```python
from build123d import *

# Parameters (mm, degrees)
F0_W     = 209.55
F0_H     = 165.1
F1_DEPTH = 3.175
F2_W     = 6.35
F2_H     = 38.1
F2_W_2   = 38.1
F2_H_2   = 6.35
F3_DEPTH = 25.4
F4_W     = 25.4
F4_H     = 50.8
F4_W_2   = 38.1
F5_DEPTH = 25.4


# Not quite as in the source:
# - a length typed as a fraction of an inch, garbled in the dataset ("3 / 203.2 mm" for 3/8 in), is restored


with BuildPart() as f1:
    # F0 (on Top) → F1 (new body)
    with BuildSketch(Plane.XY):
        Rectangle(F0_W, F0_H)
    extrude(amount=F1_DEPTH)

    # F2 (on face) → F3 (cut)
    with BuildSketch(Plane.XY.offset(3.175)):
        with Locations((-101.6, 38.1)):
            Rectangle(F2_W, F2_H)
        with Locations((-101.6, -38.1)):
            Rectangle(F2_W, F2_H)
        with Locations((101.6, 38.1)):
            Rectangle(F2_W, F2_H)
        with Locations((101.6, -38.1)):
            Rectangle(F2_W, F2_H)
        with Locations((-41.275, -79.375)):
            Rectangle(F2_W_2, F2_H_2)
        with Locations((41.275, -79.375)):
            Rectangle(F2_W_2, F2_H_2)
        with Locations((41.275, 79.375)):
            Rectangle(F2_W_2, F2_H_2)
        with Locations((-41.275, 79.375)):
            Rectangle(F2_W_2, F2_H_2)
    extrude(amount=-F3_DEPTH, mode=Mode.SUBTRACT)

    # F4 (on face) → F5 (cut)
    with BuildSketch(Plane.XY.offset(3.175)):
        with Locations((-79.375, -44.45)):
            Rectangle(F4_W, F4_H)
        with Locations((79.375, -44.45)):
            Rectangle(F4_W, F4_H)
        with Locations((0, -44.45)):
            Rectangle(F4_W_2, F4_H)
    extrude(amount=-F5_DEPTH, mode=Mode.SUBTRACT)


solid = f1.part
```
Here's how the part is built. I have some questions about the finished solid (model axes, mm). Coordinates: 2 decimals unless noted, no trailing zeros. Order: outer loops, then holes, each group sorted by start corner. A loop starts at its lowest first (then second) coordinate and runs counter-clockwise, first axis right, second up.
Item 1: If we section it at B-B, the plane z = 1: Give the number of separate pieces and of enclosed holes in the cut face, then the cut area to 3 significant figures.
Response values:
separate pieces: 1
enclosed holes: 3
area: 28,100 mm2
Item 2: If we section it at D-D, the plane x = -57: List the corners of the cut face in (y, z) for me (3 decimals).
Response values:
outline: (-76.2, 0) - (76.2, 0) - (76.2, 3.175) - (-76.2, 3.175) - close
Item 3: If we section it at A-A, the plane y = -64.5: List the corners of the cut face in (x, z) for me (3 decimals), then the cut area to 3 significant figures.
Response values:
outline: (-104.775, 0) - (-92.075, 0) - (-92.075, 3.175) - (-104.775, 3.175) - close; (-66.675, 0) - (-19.05, 0) - (-19.05, 3.175) - (-66.675, 3.175) - close; (19.05, 0) - (66.675, 0) - (66.675, 3.175) - (19.05, 3.175) - close; (92.075, 0) - (104.775, 0) - (104.775, 3.175) - (92.075, 3.175) - close
area: 383 mm2
Item 4: I need wall thicknesses on probe 1 along X at (y, z) = (-48, 2.4) (3 decimals); probe 2 along X at (y, z) = (-65.5, 1.9) (3 decimals); probe 3 along Y at (x, z) = (18, 0.4). Which ranges of each line are inside material? Lowest first, please.
Response values:
probe 1: x = -98.425 to -92.075, -66.675 to -19.05, 19.05 to 66.675, 92.075 to 98.425
probe 2: x = -104.775 to -92.075, -66.675 to -19.05, 19.05 to 66.675, 92.075 to 104.775
probe 3: y = -82.55 to -69.85, -19.05 to 82.55
Item 5: If we section it at C-C, the plane y = -36: List the corners of the cut face in (x, z) for me (3 decimals).
Response values:
outline: (-98.425, 0) - (-92.075, 0) - (-92.075, 3.175) - (-98.425, 3.175) - close; (-66.675, 0) - (-19.05, 0) - (-19.05, 3.175) - (-66.675, 3.175) - close; (19.05, 0) - (66.675, 0) - (66.675, 3.175) - (19.05, 3.175) - close; (92.075, 0) - (98.425, 0) - (98.425, 3.175) - (92.075, 3.175) - close
Item 6: I'm going to push flat-ended pins straight in: pin 1 Ø1 at (y, z) = (-56.5, 1) entering from -X (3 decimals); pin 2 Ø1 at (y, z) = (-33, 1) entering from +X (3 decimals); pin 3 Ø1 at (x, z) = (-39, 1) entering from -Y. Where does each tip first touch, or does it pass through?
Response values:
pin 1: stops at x = -98.425
pin 2: stops at x = 98.425
pin 3: stops at y = -76.2
